Read the model definition and answer for the solid it produces. Units are mm, in the model's axes. A direction names the side the tool comes from. Give positions to 0.01 mm unless a question says otherwise; leave off trailing zeros. Loops run counter-clockwise (first coordinate to the right, second up) from the corner with the lowest first, then second, coordinate; pieces in that order, holes last. Notation, with made-up numbers: (-3, 68) -> (20, 68) arc R18 cw to (20, 83) -> close; hole circle Ø8 at (24.5, 31). An arc over 180 degrees is marked (long way). One line per item, written item: value. Start each with the question number.
from build123d import *

# Parameters (mm, degrees)
SKETCH1_W           = 32
SKETCH1_H           = 28.6
SKETCH1_R           = 2.5
SKETCH1_H_2         = 30.2
SKETCH1_R_2         = 1.45
BOSS_EXTRUDE1_DEPTH = 6
BOSS_EXTRUDE2_START = 3
SKETCH1_4_W         = 32
SKETCH1_4_H         = 28.6
SKETCH1_4_R         = 2.5
SKETCH1_4_H_2       = 30.2
SKETCH1_4_R_2       = 1.45
BOSS_EXTRUDE2_DEPTH = 3
BOSS_EXTRUDE3_START = 3
SKETCH1_5_W         = 32
SKETCH1_5_H         = 28.6
SKETCH1_5_R         = 2.5
SKETCH1_5_R_2       = 1.45
BOSS_EXTRUDE3_DEPTH = 30.2
CUT_EXTRUDE1_DEPTH  = 48.647455336
CUT_EXTRUDE2_START  = -18
CUT_EXTRUDE2_DEPTH  = 30.647455336
CUT_EXTRUDE3_START  = 26
SKETCH1_6_R         = 2.5
SKETCH1_6_R_2       = 1.45
CUT_EXTRUDE3_DEPTH  = 7.2
FILLET1_R           = 0.5
CHAMFER1_SIZE       = 0.4


with BuildPart() as part:
    # Sketch1 → Boss-Extrude1 (new body)
    # profile 1 of 6: a face of its own
    with BuildSketch(Plane.YZ):
        with Locations((0, 15.1)):
            Rectangle(SKETCH1_W, SKETCH1_H)
        with Locations((-12.5, 12.5)):
            Circle(SKETCH1_R, mode=Mode.SUBTRACT)
        with Locations((12.5, 12.5)):
            Circle(SKETCH1_R, mode=Mode.SUBTRACT)
    # profile 2 of 6: a face of its own
    with BuildSketch(Plane.YZ):
        with Locations((0, -14.3)):
            Rectangle(SKETCH1_W, SKETCH1_H_2)
        with Locations((-12.5, -12.5)):
            Circle(SKETCH1_R, mode=Mode.SUBTRACT)
        with Locations((12.5, -12.5)):
            Circle(SKETCH1_R, mode=Mode.SUBTRACT)
    # profile 3 of 6: a face of its own
    with BuildSketch(Plane.YZ):
        with Locations((-12.5, 12.5)):
            Circle(SKETCH1_R)
        with Locations(Location((-12.5, 12.5, 0), (0, 0, 270))):
            Circle(SKETCH1_R_2, mode=Mode.SUBTRACT)
    # profile 4 of 6: a face of its own
    with BuildSketch(Plane.YZ):
        with Locations((12.5, 12.5)):
            Circle(SKETCH1_R)
        with Locations(Location((12.5, 12.5, 0), (0, 0, 270))):
            Circle(SKETCH1_R_2, mode=Mode.SUBTRACT)
    # profile 5 of 6: a face of its own
    with BuildSketch(Plane.YZ):
        with Locations((12.5, -12.5)):
            Circle(SKETCH1_R)
        with Locations(Location((12.5, -12.5, 0), (0, 0, 270))):
            Circle(SKETCH1_R_2, mode=Mode.SUBTRACT)
    # profile 6 of 6: a face of its own
    with BuildSketch(Plane.YZ):
        with Locations((-12.5, -12.5)):
            Circle(SKETCH1_R)
        with Locations(Location((-12.5, -12.5, 0), (0, 0, 270))):
            Circle(SKETCH1_R_2, mode=Mode.SUBTRACT)
    extrude(amount=-BOSS_EXTRUDE1_DEPTH)

    # Sketch1<4> → Boss-Extrude2 (add)
    # profile 1 of 4: a face of its own
    with BuildSketch(Plane.YZ.offset(BOSS_EXTRUDE2_START)):
        with Locations((0, 15.1)):
            Rectangle(SKETCH1_4_W, SKETCH1_4_H)
        with Locations((-12.5, 12.5)):
            Circle(SKETCH1_4_R, mode=Mode.SUBTRACT)
        with Locations((12.5, 12.5)):
            Circle(SKETCH1_4_R, mode=Mode.SUBTRACT)
    # profile 2 of 4: a face of its own
    with BuildSketch(Plane.YZ.offset(BOSS_EXTRUDE2_START)):
        with Locations((0, -14.3)):
            Rectangle(SKETCH1_4_W, SKETCH1_4_H_2)
        with Locations(Location((-12.5, -12.5, 0), (0, 0, 270))):
            Circle(SKETCH1_4_R, mode=Mode.SUBTRACT)
        with Locations(Location((12.5, -12.5, 0), (0, 0, 270))):
            Circle(SKETCH1_4_R, mode=Mode.SUBTRACT)
    # profile 3 of 4: a face of its own
    with BuildSketch(Plane.YZ.offset(BOSS_EXTRUDE2_START)):
        with Locations((12.5, 12.5)):
            Circle(SKETCH1_4_R)
        with Locations(Location((12.5, 12.5, 0), (0, 0, 270))):
            Circle(SKETCH1_4_R_2, mode=Mode.SUBTRACT)
    # profile 4 of 4: a face of its own
    with BuildSketch(Plane.YZ.offset(BOSS_EXTRUDE2_START)):
        with Locations((-12.5, 12.5)):
            Circle(SKETCH1_4_R)
        with Locations(Location((-12.5, 12.5, 0), (0, 0, 270))):
            Circle(SKETCH1_4_R_2, mode=Mode.SUBTRACT)
    extrude(amount=-BOSS_EXTRUDE2_DEPTH)

    # Sketch1<5> → Boss-Extrude3 (add)
    # profile 1 of 3: a face of its own
    with BuildSketch(Plane.YZ.offset(BOSS_EXTRUDE3_START)):
        with Locations((0, 15.1)):
            Rectangle(SKETCH1_5_W, SKETCH1_5_H)
        with Locations((-12.5, 12.5)):
            Circle(SKETCH1_5_R, mode=Mode.SUBTRACT)
        with Locations((12.5, 12.5)):
            Circle(SKETCH1_5_R, mode=Mode.SUBTRACT)
    # profile 2 of 3: a face of its own
    with BuildSketch(Plane.YZ.offset(BOSS_EXTRUDE3_START)):
        with Locations((-12.5, 12.5)):
            Circle(SKETCH1_5_R)
        with Locations(Location((-12.5, 12.5, 0), (0, 0, 270))):
            Circle(SKETCH1_5_R_2, mode=Mode.SUBTRACT)
    # profile 3 of 3: a face of its own
    with BuildSketch(Plane.YZ.offset(BOSS_EXTRUDE3_START)):
        with Locations((12.5, 12.5)):
            Circle(SKETCH1_5_R)
        with Locations(Location((12.5, 12.5, 0), (0, 0, 270))):
            Circle(SKETCH1_5_R_2, mode=Mode.SUBTRACT)
    extrude(amount=BOSS_EXTRUDE3_DEPTH)

    # Sketch2 → Cut-Extrude1 (cut, through all)
    with BuildSketch(Plane(origin=(0, 0, 0.8), x_dir=(1, 0, 0), z_dir=(0, 0, -1))):
        with BuildLine():
            ThreePointArc((21.4, 0), (20.4627417, 2.2627417), (18.2, 3.2))
            Line((18.2, 3.2), (18.2, -3.2))
            ThreePointArc((18.2, -3.2), (20.4627417, -2.2627417), (21.4, 0))
        make_face()
        with BuildLine():
            Line((18.2, -3.2), (18.2, 3.2))
            ThreePointArc((18.2, 3.2), (15, 0), (18.2, -3.2))
        make_face()
    extrude(amount=-CUT_EXTRUDE1_DEPTH, mode=Mode.SUBTRACT)

    # Sketch2<3> → Cut-Extrude2 (cut, through all)
    with BuildSketch(Plane(origin=(0, 0, 0.8), x_dir=(1, 0, 0), z_dir=(0, 0, -1)).offset(CUT_EXTRUDE2_START)):
        with BuildLine():
            ThreePointArc((24.2, 0), (22.442640687, 4.242640687), (18.2, 6))
            Line((18.2, 6), (18.2, 3.2))
            ThreePointArc((18.2, 3.2), (20.4627417, 2.2627417), (21.4, 0))
            ThreePointArc((21.4, 0), (20.4627417, -2.2627417), (18.2, -3.2))
            Line((18.2, -3.2), (18.2, -6))
            ThreePointArc((18.2, -6), (22.442640687, -4.242640687), (24.2, 0))
        make_face()
        with BuildLine():
            Line((18.2, 3.2), (18.2, 6))
            ThreePointArc((18.2, 6), (12.2, 0), (18.2, -6))
            Line((18.2, -6), (18.2, -3.2))
            ThreePointArc((18.2, -3.2), (15, 0), (18.2, 3.2))
        make_face()
    extrude(amount=-CUT_EXTRUDE2_DEPTH, mode=Mode.SUBTRACT)

    # Sketch1<6> → Cut-Extrude3 (cut)
    # profile 1 of 2: a face of its own
    with BuildSketch(Plane.YZ.offset(CUT_EXTRUDE3_START)):
        with Locations(Location((-12.5, 12.5, 0), (0, 0, 90))):
            Circle(SKETCH1_6_R)
        with Locations(Location((-12.5, 12.5, 0), (0, 0, 270))):
            Circle(SKETCH1_6_R_2, mode=Mode.SUBTRACT)
    # profile 2 of 2: a face of its own
    with BuildSketch(Plane.YZ.offset(CUT_EXTRUDE3_START)):
        with Locations(Location((12.5, 12.5, 0), (0, 0, 90))):
            Circle(SKETCH1_6_R)
        with Locations(Location((12.5, 12.5, 0), (0, 0, 270))):
            Circle(SKETCH1_6_R_2, mode=Mode.SUBTRACT)
    extrude(amount=CUT_EXTRUDE3_DEPTH, mode=Mode.SUBTRACT)

    # Fillet1
    fillet1_edges = [part.edges().sort_by_distance(p)[0] for p in [
        (13.6, -16, 29.4),
        (13.6, 16, 29.4),
        (-1.5, 16, -29.4),
        (-1.5, -16, -29.4),
        (18.1, -16, 0.8),
        (18.1, 16, 0.8),
    ]]
    fillet(fillet1_edges, radius=FILLET1_R)

    # Chamfer1
    chamfer1_edges = [part.edges().sort_by_distance(p)[0] for p in [
        (3, 16, -13.8),
        (-6, 16, 0),
        (33.2, -16, 15.1),
        (33.2, 0, 0.8),
        (0, -12.5, -11.05),
        (33.2, 0, 29.4),
        (33.2, -15.853553391, 0.946446609),
        (33.2, 15.853553391, 0.946446609),
        (33.2, -15.853553391, 29.253553391),
        (33.2, 15.853553391, 29.253553391),
        (-6, 0, 29.4),
        (0, 12.5, -11.05),
        (-6, -16, 0),
        (-6, 0, -29.4),
        (-6, -15.853553391, -29.253553391),
        (-6, 15.853553391, -29.253553391),
        (-6, -15.853553391, 29.253553391),
        (-6, 15.853553391, 29.253553391),
        (3, -16, -13.8),
        (3, 0, -29.4),
        (3, -15.853553391, -29.253553391),
        (3, 15.853553391, -29.253553391),
        (-6, -12.5, 13.95),
        (3, 12.5, -10),
        (3, -12.5, -10),
        (-6, 12.5, 13.95),
        (-6, 12.5, -11.05),
        (-6, -12.5, -11.05),
        (18.2, 3.2, 0.8),
        (18.2, 3.2, 18.8),
        (18.2, 6, 29.4),
        (33.2, -12.5, 10),
        (26, -12.5, 13.95),
        (33.2, 12.5, 10),
        (26, 12.5, 13.95),
        (33.2, 16, 15.1),
    ]]
    chamfer(chamfer1_edges, length=CHAMFER1_SIZE)


solid = part.part
Item 1: Consider L1, parallel to Y at x = 29, z = 12.5; L2, parallel to Y at x = -4, z = -12; L3, parallel to X at y = -10, z = -0.5. Determine where each line is inside the solid, lowest interval first. Write a range as [from, to].
Item 2: For faces 1 (the cylindrical face through (10.22, -13.38, 13.65)), 2 (the cylindrical face through (1.32, 10.06, -11.96)), 3 (the flat face through (14, 0, 0.8)), determine the directions among +Z, -Z, +X, -X, +Y, -Y from which every point of the face is accessible in a straight line to the end or side of a thin tool.
Item 3: Section A-A, the plane z = 26 is taken. Determine the outline of the cut face in (x, y).
Item 4: Determine the mould class of faces 4 (the cylindrical face through (29.35, -10.06, 11.96)), 5 (the flat face through (33.2, 0, 15)) for opening direction Y: pulls with the +Y half, pulls with the -Y half, needs draft (parallel to the pull), parting line crosses it, or undercut.
Item 5: Section D-D, the plane y = 12.5 is taken. State how many separate pieces and enclosed holes the cut face has, plus the area to 3 significant figures.
Item 6: Flat-ended cylindrical pins translate along their axes: pin 1 (3.5 mm diameter, centred on y = -12.5, z = -12.5, fed in from +X); pin 2 (3.5 mm diameter, centred on x = 16.5, y = -0.5, fed in from +Z); pin 3 (2.5 mm diameter, centred on y = -12.5, z = 13, fed in from +X). Find the tip coordinate at first contact, or state that the pin passes through.
Item 7: Section B-B, the plane x = 9.5 is taken. Determine the outline of the cut face in (y, z), plus the area to 3 significant figures.
Item 8: Section C-C, the plane z = -1 is taken. Determine the outline of the cut face in (x, y).
Computed values:
1. L1: [-16, -15], [-10, 10], [15, 16]
1. L2: [-16, -13.86], [-11.14, 11.14], [13.86, 16]
1. L3: [-6, 3]
2. face 1: +X, -X
2. face 2: +X
2. face 3: -Z, +X, +Y, -Y
3. outline: (-6, -15.6) -> (-5.6, -16) -> (32.8, -16) -> (33.2, -15.6) -> (33.2, 15.6) -> (32.8, 16) -> (-5.6, 16) -> (-6, 15.6) -> close; hole circle Ø12 at (18.2, 0)
4. face 4: undercut
4. face 5: needs draft
5. separate pieces: 3
5. enclosed holes: 0
5. area: 1,230 mm²
6. pin 1: x = -0.1
6. pin 2: z = 18.72
6. pin 3: x = 25.9
7. outline: (-16, 1.3) arc R0.5 ccw to (-15.5, 0.8) -> (15.5, 0.8) arc R0.5 ccw to (16, 1.3) -> (16, 28.9) arc R0.5 ccw to (15.5, 29.4) -> (-15.5, 29.4) arc R0.5 ccw to (-16, 28.9) -> close; hole circle Ø2.9 at (-12.5, 12.5); hole circle Ø2.9 at (12.5, 12.5)
7. area: 902 mm²
8. outline: (-6, -15.6) -> (-5.6, -16) -> (2.6, -16) -> (3, -15.6) -> (3, 15.6) -> (2.6, 16) -> (-5.6, 16) -> (-6, 15.6) -> close
